Check sheet for the modelled part. Datum: model origin and axes. Units: mm. Round coordinates to 2 decimals unless told otherwise and drop trailing zeros. Loops run counter-clockwise (first coordinate to the right, second up) from the corner with the lowest first, then second, coordinate; pieces in that order, holes last. Notation, with made-up numbers: (65.5, 2.5) -> (86.5, 2.5) arc R14 cw to (86.5, 27.5) -> close; hole circle Ø8 at (19, 26.5). An arc over 180 degrees is marked (long way). Return JSON: item names as keys, results as strings.
from build123d import *

# Parameters (mm, degrees)
SKETCH1_W           = 236
SKETCH1_H           = 366
BOSS_EXTRUDE1_DEPTH = 3
CUT_EXTRUDE2_REACH  = 5
SKETCH2_R           = 7.5
CUT_EXTRUDE3_REACH  = 5
SKETCH3_R           = 11
SKETCH3_R_2         = 10


with BuildPart() as part:
    # Sketch1 → Boss-Extrude1 (new body)
    with BuildSketch(Plane.XY):
        Rectangle(SKETCH1_W, SKETCH1_H)
    extrude(amount=BOSS_EXTRUDE1_DEPTH)

    # Sketch2 → Cut-Extrude2 (cut, up to next)
    with BuildSketch(Plane(origin=(0, 0, 0), x_dir=(-1, 0, 0), z_dir=(0, 0, -1)), mode=Mode.PRIVATE) as cut_extrude2_sk1:
        with Locations((0, 137.5)):
            Circle(SKETCH2_R)
    cut_extrude2_tool1 = extrude(cut_extrude2_sk1.sketch, amount=-CUT_EXTRUDE2_REACH, mode=Mode.PRIVATE) & part.part
    add(cut_extrude2_tool1.solids().sort_by_distance((0, 137.5, 0))[0], mode=Mode.SUBTRACT)

    # Sketch3 → Cut-Extrude3 (cut, up to next)
    with BuildSketch(Plane.XY.offset(3), mode=Mode.PRIVATE) as cut_extrude3_sk1:
        Circle(SKETCH3_R)
    cut_extrude3_tool1 = extrude(cut_extrude3_sk1.sketch, amount=-CUT_EXTRUDE3_REACH, mode=Mode.PRIVATE) & part.part
    add(cut_extrude3_tool1.solids().sort_by_distance((0, 0, 3))[0], mode=Mode.SUBTRACT)
    # Sketch3 → Cut-Extrude3 (cut, up to next)
    with BuildSketch(Plane.XY.offset(3), mode=Mode.PRIVATE) as cut_extrude3_sk2:
        with Locations((-58.75, -62.75)):
            Circle(SKETCH3_R_2)
    cut_extrude3_tool2 = extrude(cut_extrude3_sk2.sketch, amount=-CUT_EXTRUDE3_REACH, mode=Mode.PRIVATE) & part.part
    add(cut_extrude3_tool2.solids().sort_by_distance((-58.75, -62.75, 3))[0], mode=Mode.SUBTRACT)
    # Sketch3 → Cut-Extrude3 (cut, up to next)
    with BuildSketch(Plane.XY.offset(3), mode=Mode.PRIVATE) as cut_extrude3_sk3:
        with Locations((58.75, -62.75)):
            Circle(SKETCH3_R_2)
    cut_extrude3_tool3 = extrude(cut_extrude3_sk3.sketch, amount=-CUT_EXTRUDE3_REACH, mode=Mode.PRIVATE) & part.part
    add(cut_extrude3_tool3.solids().sort_by_distance((58.75, -62.75, 3))[0], mode=Mode.SUBTRACT)
    # Sketch3 → Cut-Extrude3 (cut, up to next)
    with BuildSketch(Plane.XY.offset(3), mode=Mode.PRIVATE) as cut_extrude3_sk4:
        with Locations((0, 137.015625)):
            Circle(SKETCH3_R_2)
    cut_extrude3_tool4 = extrude(cut_extrude3_sk4.sketch, amount=-CUT_EXTRUDE3_REACH, mode=Mode.PRIVATE) & part.part
    add(cut_extrude3_tool4.solids().sort_by_distance((0, 137.015625, 3))[0], mode=Mode.SUBTRACT)


solid = part.part
Q1. Section check A-A (x = 58.75). Record the boundary of the cut face in (y, z).
Results list:
{"outline": "(-183, 0) -> (-72.75, 0) -> (-72.75, 3) -> (-183, 3) -> close; (-52.75, 0) -> (183, 0) -> (183, 3) -> (-52.75, 3) -> close"}
Q2. Section check C-C (y = 0). Record the boundary of the cut face in (x, z), then the cut area to 3 significant figures.
Results list:
{"outline": "(-118, 0) -> (-11, 0) -> (-11, 3) -> (-118, 3) -> close; (11, 0) -> (118, 0) -> (118, 3) -> (11, 3) -> close", "area": "642 mm^2"}
Q3. Section check B-B (y = -62.75). Record the boundary of the cut face in (x, z), then the cut area to 3 significant figures.
Results list:
{"outline": "(-118, 0) -> (-68.75, 0) -> (-68.75, 3) -> (-118, 3) -> close; (-48.75, 0) -> (48.75, 0) -> (48.75, 3) -> (-48.75, 3) -> close; (68.75, 0) -> (118, 0) -> (118, 3) -> (68.75, 3) -> close", "area": "588 mm^2"}
Q4. Draft check along Y on faces 1 (the cylindrical face through (50.81, -68.83, 1.52)), 2 (the flat face through (-28, 3, 0)). Enter one of: released by +Y, released by -Y, zero draft, split by the parting line, or undercut.
Results list:
{"face 1": "undercut", "face 2": "zero draft"}
Q5. Section check D-D (x = 0). Record the boundary of the cut face in (y, z), then the cut area to 3 significant figures.
Results list:
{"outline": "(-183, 0) -> (-11, 0) -> (-11, 3) -> (-183, 3) -> close; (11, 0) -> (127.02, 0) -> (127.02, 3) -> (11, 3) -> close; (147.02, 0) -> (183, 0) -> (183, 3) -> (147.02, 3) -> close", "area": "972 mm^2"}
Q6. Go/stop test with a flat-tipped pin: pin 1 (13 mm diameter, centred on x = 0, y = 0, fed in from -Z). Record where the tip stops, or that it passes through.
Results list:
{"pin 1": "through"}
Q7. Material ranges on line 1 (Y direction, x = -58.75, z = 0.9); line 2 (X direction, y = -59.5, z = 2.45); line 3 (Y direction, x = -8.5, z = 0.5), recorded low to high.
Results list:
{"line 1": "-183 to -72.75, -52.75 to 183", "line 2": "-118 to -68.21, -49.29 to 49.29, 68.21 to 118", "line 3": "-183 to -6.98, 6.98 to 131.75, 142.28 to 183"}
